Part model, mm, in its own coordinate system. A direction names the side the tool comes from. Coordinates: 2 decimals unless noted, no trailing zeros. Loops run counter-clockwise (first coordinate to the right, second up) from the corner with the lowest first, then second, coordinate; pieces in that order, holes last. Notation, with made-up numbers: (67.5, 21) -> (93.5, 21) arc R13 ccw to (93.5, 25) -> close; hole circle Ø10 at (14.25, 50). An arc over 180 degrees is marked (long way). One line per question, with ' | ' between items. Start each with the question number.
1) Cut at D-D (x = 9.5). List the corners of the cut face in (y, z).
2) Cut at C-C (x = -4). List the corners of the cut face in (y, z).
3) Cut at B-B (z = -16.25). List the corners of the cut face in (x, y), plus the area to 3 significant figures.
4) Drop flat-ended pins along their axis: pin 1 (12 mm diameter, centred on x = 6.5, z = -39, fed in from +Y); pin 2 (7.5 mm diameter, centred on x = 3.5, y = -15.5, fed in from -Z); pin 3 (2 mm diameter, centred on x = -18, y = 1.5, fed in from -Z); pin 4 (2.5 mm diameter, centred on x = 0, z = -16.25, fed in from +Y). Give the stop position or say it passes through.
5) Two-plate mould, pull along Z, no slides. Class faces 1 (the face through (0, 0, -23)), 2 (the face through (0.559, 9.7, -57.144)), 3 (the face through (-11.936, 1.288, -24.195)): released by +Z, released by -Z, zero draft, split by the parting line, or undercut.
6) Cut at A-A (y = 19.5). List the corners of the cut face in (x, z), plus the area to 3 significant figures.
7) 3-axis set-ups, long thin cutter, end or side, ignore diameter. For faces 4 (the face through (-18.888, 11.59, -34.23)), 5 (the face through (13.5, 1.3, -41)), 6 (the face through (0, -10, 0)): which of +Z, -Z, +X, -X, +Y, -Y reach the whole face in a straight line?
8) Probe L1, parallel to Z at x = -1.5, y = -8.5; L2, parallel to Y at x = -14.5, z = -44; L3, parallel to X at y = 1.35, z = -39.5. List the from-to ranges inside material, lowest first. Write a range as from..to.
from build123d import *

# Parameters (mm, degrees)
SKETCH1_R           = 25.4
BOSS_EXTRUDE1_DEPTH = 12.7
SKETCH2_R           = 25.4
SKETCH2_W           = 50.8
SKETCH2_H           = 31.75
BOSS_EXTRUDE2_DEPTH = 25.4
SKETCH4_R           = 19.05
CUT_EXTRUDE2_DEPTH  = 22.86
CUT_EXTRUDE1_DEPTH  = 68.501425911
SKETCH5_R           = 7.62
SKETCH5_R_2         = 1.5
CUT_EXTRUDE3_DEPTH  = 69.497635846


with BuildPart() as part:
    # Sketch1 → Boss-Extrude1 (new body)
    with BuildSketch(Plane.XY):
        Circle(SKETCH1_R)
    extrude(amount=BOSS_EXTRUDE1_DEPTH)

    # Sketch2 → Boss-Extrude2 (add)
    with BuildSketch(Plane(origin=(0, 0, 0), x_dir=(1, 0, 0), z_dir=(0, 1, 0))):
        with Locations((0, 31.75)):
            Circle(SKETCH2_R)
        with Locations((0, 15.875)):
            Rectangle(SKETCH2_W, SKETCH2_H)
    extrude(amount=BOSS_EXTRUDE2_DEPTH)

    # Sketch4 → Cut-Extrude2 (cut)
    with BuildSketch(Plane.XZ.offset(-25.4)):
        with Locations(Location((0, -31.75, 0), (0, 0, 90))):
            Circle(SKETCH4_R)
    extrude(amount=CUT_EXTRUDE2_DEPTH, mode=Mode.SUBTRACT)

    # Sketch3 → Cut-Extrude1 (cut, through all)
    with BuildSketch(Plane.XY):
        with BuildLine():
            ThreePointArc((0, 25.4), (17.960512242, 17.960512242), (25.4, 0))
            Line((25.4, 0), (25.4, 25.4))
            Line((25.4, 25.4), (0, 25.4))
        make_face()
        with BuildLine():
            ThreePointArc((-25.4, 0), (-17.960512242, 17.960512242), (0, 25.4))
            Line((0, 25.4), (-25.4, 25.4))
            Line((-25.4, 25.4), (-25.4, 0))
        make_face()
    extrude(amount=-CUT_EXTRUDE1_DEPTH, mode=Mode.SUBTRACT)

    # Sketch5 → Cut-Extrude3 (cut, through all)
    with BuildSketch(Plane(origin=(0, 2.54, 0), x_dir=(1, 0, 0), z_dir=(0, 1, 0))):
        with Locations(Location((0, 31.75, 0), (0, 0, 270))):
            Circle(SKETCH5_R)
        with Locations(Location((0, 47.249999988, 0), (0, 0, 270))):
            Circle(SKETCH5_R_2)
        with Locations(Location((13.423393748, 39.499999994, 0), (0, 0, 270))):
            Circle(SKETCH5_R_2)
        with Locations(Location((13.423393748, 24.000000006, 0), (0, 0, 270))):
            Circle(SKETCH5_R_2)
        with Locations(Location((0, 16.250000012, 0), (0, 0, 270))):
            Circle(SKETCH5_R_2)
        with Locations(Location((-13.423393748, 24.000000006, 0), (0, 0, 270))):
            Circle(SKETCH5_R_2)
        with Locations(Location((-13.423393748, 39.499999994, 0), (0, 0, 270))):
            Circle(SKETCH5_R_2)
    extrude(amount=-CUT_EXTRUDE3_DEPTH, mode=Mode.SUBTRACT)


solid = part.part
Reported:
1) outline: (-23.56, 0) -> (0, 0) -> (0, -55.31) -> (23.56, -55.31) -> (23.56, -48.26) -> (2.54, -48.26) -> (2.54, -15.24) -> (23.56, -15.24) -> (23.56, 12.7) -> (-23.56, 12.7) -> close
2) outline: (-25.08, 0) -> (0, 0) -> (0, -25.26) -> (2.54, -25.26) -> (2.54, -13.12) -> (25.08, -13.12) -> (25.08, 12.7) -> (-25.08, 12.7) -> close; (0, -56.83) -> (25.08, -56.83) -> (25.08, -50.38) -> (2.54, -50.38) -> (2.54, -38.24) -> (0, -38.24) -> close
3) outline: (-25.4, 0) -> (-1.5, 0) -> (-1.5, 2.54) -> (-11.07, 2.54) -> (-11.07, 22.86) arc R25.4 ccw to start; (1.5, 0) -> (25.4, 0) arc R25.4 ccw to (11.07, 22.86) -> (11.07, 2.54) -> (1.5, 2.54) -> close | area: 518 mm²
4) pin 1: stops at y = 2.54 | pin 2: stops at z = 0 | pin 3: stops at z = -50.62 | pin 4: passes through
5) face 1: zero draft | face 2: released by -Z | face 3: undercut
6) outline: (-16.28, -51.25) arc R25.4 ccw to (16.28, -51.25) -> (16.28, -41.65) arc R19.05 cw to (-16.28, -41.65) -> close; (-16.28, -21.85) arc R19.05 cw to (16.28, -21.85) -> (16.28, 12.7) -> (-16.28, 12.7) -> close | area: 1,150 mm²
7) face 4: +Y | face 5: +Y, -Y | face 6: -Z, +X, -X, -Y
8) L1: z = 0..12.7 | L2: y = 0..2.54 | L3: x = -24.19..-14.92, -11.92..11.92, 14.92..24.19
